```python
from build123d import *

# Parameters (mm, degrees)
SKETCH1_W                   = 106
SKETCH1_H                   = 46
BOSS_EXTRUDE1_DEPTH         = 6
M5_CLEARANCE_HOLE1_D        = 5.5
TAP_DRILL_FOR_M3X0_5_TAP1_D = 2.5


with BuildPart() as part:
    # Sketch1 → Boss-Extrude1 (new body)
    with BuildSketch(Plane(origin=(0, 0, 0), x_dir=(1, 0, 0), z_dir=(0, 1, 0))):
        with Locations((-19.22561214, 10.934191123)):
            Rectangle(SKETCH1_W, SKETCH1_H)
    extrude(amount=-BOSS_EXTRUDE1_DEPTH)

    # M5 Clearance Hole1 (through all)
    with Locations(Plane(origin=(-56.72561214, 0, -18.384191123), x_dir=(0, 0, 1), z_dir=(0, 1, 0))):
        with Locations((0, 0), (0, 25), (0, 50), (0, 75), (14.9, 75), (14.9, 50), (14.9, 25), (14.9, 0)):
            Hole(M5_CLEARANCE_HOLE1_D / 2)

    # Tap Drill for M3x0.5 Tap1 (through all)
    with Locations(Plane(origin=(-63.39561214, 0, 0.565808877), x_dir=(0, 0, 1), z_dir=(0, 1, 0))):
        with Locations((0, 0), (0, 8.83), (0, 26.49), (0, 35.32), (0, 52.98), (0, 44.15), (0, 17.66), (0, 61.81), (0, 70.64), (0, 79.47), (0, 88.3), (-23, 88.3), (-23, 79.47), (-23, 70.64), (-23, 61.81), (-23, 52.98), (-23, 44.15), (-23, 35.32), (-23, 26.49), (-23, 17.66), (-23, 8.83), (-23, 0), (-11.5, 0), (-11.5, 8.83), (-11.5, 17.66), (-11.5, 26.49), (-11.5, 52.98), (-11.5, 61.81), (-11.5, 79.47), (-11.5, 88.3), (-11.5, 35.32), (-11.5, 70.64), (-11.5, 44.15)):
            Hole(TAP_DRILL_FOR_M3X0_5_TAP1_D / 2)


solid = part.part
```
Can you work these out from the model? Positions are in its coordinate system, mm. Round coordinates to 2 decimals unless told otherwise and drop trailing zeros. Loops run counter-clockwise (first coordinate to the right, second up) from the corner with the lowest first, then second, coordinate; pieces in that order, holes last. Notation, with made-up numbers: (56, -15) -> (115, -15) arc R15 cw to (115, -1) -> close; hole circle Ø9 at (28.25, -11). An arc over 180 degrees is marked (long way). One line per item, written item: value. Start each with the question number.
1. If I drill on probe 1 along X at (y, z) = (-5.6, -2); probe 2 along X at (y, z) = (-3.35, -20.5), over which ranges is the centre line in solid material (lowest first)?
2. If we section it at A-A, the plane z = -5: Write out the boundary of the cut face in (x, y), then the cut area to 3 significant figures.
3. If we mould it in two halves opening along X, with no side actions, what happens to faces 1 (the cylindrical face through (16.919, -3.042, -21.513)), 2 (the flat face through (33.774, -3, -11))? For each: pulls with the +X half, pulls with the -X half, needs draft (parallel to the pull), parting line crosses it, or undercut.
4. For pin 1 (2 mm diameter, centred on x = 24.9, z = -22.43, fed in from -Y), with a flat end and sliding along its axis, tell me the tip position at first contact or that it passes through.
5. If we section it at B-B, the plane y = -4.95: Give the number of separate pieces and of enclosed holes in the cut face, then the cut area to 3 significant figures.
Calculated:
1. probe 1: x = -72.23 to -59.04, -54.41 to -34.04, -29.41 to -9.04, -4.41 to 15.96, 20.59 to 33.77
1. probe 2: x = -72.23 to -58.48, -54.97 to -33.48, -29.97 to -8.48, -4.97 to 16.52, 20.03 to 33.77
2. outline: (-72.23, -6) -> (-59.02, -6) -> (-59.02, 0) -> (-72.23, 0) -> close; (-54.43, -6) -> (-34.02, -6) -> (-34.02, 0) -> (-54.43, 0) -> close; (-29.43, -6) -> (-9.02, -6) -> (-9.02, 0) -> (-29.43, 0) -> close; (-4.43, -6) -> (15.98, -6) -> (15.98, 0) -> (-4.43, 0) -> close; (20.57, -6) -> (33.77, -6) -> (33.77, 0) -> (20.57, 0) -> close
2. area: 526 mm²
3. face 1: undercut
3. face 2: pulls with the +X half
4. pin 1: passes through
5. separate pieces: 1
5. enclosed holes: 41
5. area: 4,520 mm²
